CAD build for the part. Positions are in the model's coordinates, mm. Face numbers are marked on the shaded views. Give positions to 0.01 mm unless a question says otherwise; leave off trailing zeros. Write each loop counter-clockwise with the first axis right and the second up, starting at its lowest first coordinate (ties: lowest second). Pieces come first, ordered by that corner, then holes. Notation, with made-up numbers: M -37.75,-23 L 1.25,-23 A19 cw 1.25,-12 Z; hole C 45,-32 d11. An arc over 180 degrees is marked long. One line per question, with ' | ' between items. Start each with the question number.
1. Wall check: L1, parallel to Z at x = -60, y = 0.55; L2, parallel to Z at x = -18, y = 0.95; L3, parallel to Z at x = -71.5, y = 1.75. Give the ranges that are in metal, low to high.
2. Flat gauge pin, fed straight in: pin 1 (5 mm diameter, centred on x = -53, z = -50, fed in from +Y). Where does the tip first touch, or does it go through?
3. Pull direction X, two halves, no side cores. Call the marked faces 1, 2 and 3: released by +X, released by -X, zero draft, split by the parting line, or undercut.
4. Cut at D-D, the plane z = -37.5. Count the separate pieces of the cut face and the enclosed holes in it, then the cut area to 3 significant figures.
5. Cut at B-B, the plane x = -72. Write the cut outline in (y, z), then the cut area to 4 significant figures.
6. Cut at A-A, the plane x = -42. Write the cut outline in (y, z), then the cut area to 3 significant figures.
7. Cut at C-C, the plane y = 2.5. Write the cut outline in (x, z).
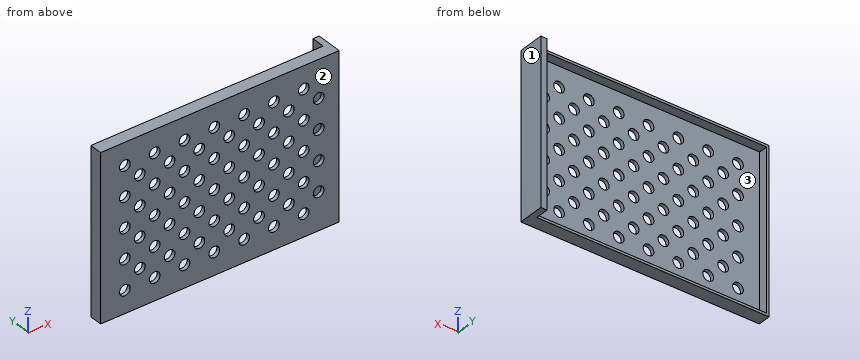
Autodesk Inventor part; units mm, degrees
ref_plane "YZ Plane" through (0, 0, 0) normal (1, 0, 0) x (0, 1, 0)
ref_plane "XZ Plane" through (0, 0, 0) normal (0, 1, 0) x (-1, 0, 0)
ref_plane "XY Plane" through (0, 0, 0) normal (0, 0, 1) x (1, 0, 0)
sketch "Sketch1" plane through (0, 0, 0) normal (0, 1, 0) x (-1, 0, 0)
  line L0 (0, 0) -> (91.5, 0)
  line L1 (91.5, 0) -> (91.5, -63)
  line L2 (91.5, -63) -> (0, -63)
  circle A0 centre (84, -7.5) radius 2.15
  circle A1 centre (84, -19.5) radius 2.15
  circle A2 centre (84, -31.5) radius 2.15
  circle A3 centre (84, -55.5) radius 2.15
  circle A4 centre (84, -43.5) radius 2.15
  circle A5 centre (78, -13.5) radius 2.15
  circle A6 centre (78, -25.5) radius 2.15
  circle A7 centre (78, -37.5) radius 2.15
  circle A8 centre (78, -49.5) radius 2.15
  circle A9 centre (66, -13.5) radius 2.15
  circle A10 centre (66, -25.5) radius 2.15
  circle A11 centre (66, -37.5) radius 2.15
  circle A12 centre (66, -49.5) radius 2.15
  circle A13 centre (72, -31.5) radius 2.15
  circle A14 centre (72, -19.5) radius 2.15
  circle A15 centre (72, -7.5) radius 2.15
  circle A16 centre (72, -55.5) radius 2.15
  circle A17 centre (72, -43.5) radius 2.15
  line L3 (66, -55.5) -> (63, -55.5)
  line L4 (63, -55.5) -> (63, -45.305)
  circle A18 centre (42, -13.5) radius 2.15
  circle A19 centre (42, -25.5) radius 2.15
  circle A20 centre (42, -37.5) radius 2.15
  circle A21 centre (42, -49.5) radius 2.15
  circle A22 centre (48, -31.5) radius 2.15
  circle A23 centre (48, -19.5) radius 2.15
  circle A24 centre (48, -7.5) radius 2.15
  circle A25 centre (48, -55.5) radius 2.15
  circle A26 centre (48, -43.5) radius 2.15
  circle A27 centre (54, -37.5) radius 2.15
  circle A28 centre (60, -31.5) radius 2.15
  circle A29 centre (54, -25.5) radius 2.15
  circle A30 centre (60, -19.5) radius 2.15
  circle A31 centre (54, -13.5) radius 2.15
  circle A32 centre (60, -7.5) radius 2.15
  circle A33 centre (60, -43.5) radius 2.15
  circle A34 centre (54, -49.5) radius 2.15
  circle A35 centre (60, -55.5) radius 2.15
  line L5 (42, -55.5) -> (39, -55.5)
  line L6 (39, -55.5) -> (39, -51.65)
  circle A36 centre (6, -37.5) radius 2.15
  circle A37 centre (12, -31.5) radius 2.15
  circle A38 centre (6, -25.5) radius 2.15
  circle A39 centre (12, -19.5) radius 2.15
  circle A40 centre (6, -13.5) radius 2.15
  circle A41 centre (12, -7.5) radius 2.15
  circle A42 centre (12, -43.5) radius 2.15
  circle A43 centre (6, -49.5) radius 2.15
  circle A44 centre (12, -55.5) radius 2.15
  line L7 (12, -55.5) -> (15, -55.5)
  line L8 (15, -55.5) -> (15, -45.305)
  circle A45 centre (36, -43.5) radius 2.15
  circle A46 centre (30, -49.5) radius 2.15
  circle A47 centre (24, -55.5) radius 2.15
  circle A48 centre (24, -43.5) radius 2.15
  circle A49 centre (36, -55.5) radius 2.15
  circle A50 centre (36, -7.5) radius 2.15
  circle A51 centre (30, -25.5) radius 2.15
  circle A52 centre (30, -13.5) radius 2.15
  circle A53 centre (18, -25.5) radius 2.15
  circle A54 centre (24, -19.5) radius 2.15
  circle A55 centre (18, -13.5) radius 2.15
  circle A56 centre (24, -7.5) radius 2.15
  circle A57 centre (36, -19.5) radius 2.15
  circle A58 centre (36, -31.5) radius 2.15
  circle A59 centre (30, -37.5) radius 2.15
  circle A60 centre (24, -31.5) radius 2.15
  circle A61 centre (18, -49.5) radius 2.15
  circle A62 centre (18, -37.5) radius 2.15
  line L9 (36, -55.5) -> (39, -55.5)
  line L10 (0, 0) -> (0, -63)
  dimension "d0" = 91.5
  dimension "d1" = 63
  dimension "d2" = 4.3
  dimension "d3" = 7.5
  dimension "d4" = 7.5
  dimension "d11" = 4.3
  dimension "d17" = 3
  dimension "d18" = 3
extrude "Extrusion1" add sketch "Sketch1" along normal blind 1.5
sketch "Sketch2" plane through (0, 1.5, 0) normal (0, 1, 0) x (1, 0, 0)
  line L0 (3, 0) -> (3, -3)
  line L1 (3, -3) -> (-94.5, -3)
  line L2 (-94.5, -3) -> (-94.5, 66)
  line L3 (-94.5, 66) -> (3, 66)
  line L4 (3, 66) -> (3, 0)
  line L5 (-91.5, 63) -> (-91.5, 0)
  line L6 (0, 63) -> (-91.5, 63)
  line L7 (-91.5, 0) -> (0, 0)
  line L8 (0, 0) -> (0, 63)
  line L9 (0, 63) -> (-91.5, 63)
  line L10 (-91.5, 63) -> (-91.5, 0)
  dimension "d30" = 97.5
  dimension "d31" = 69
  dimension "d32" = 97.5
extrude "Extrusion2" add sketch "Sketch2" along normal blind 3.612 and the other way blind 1.5
sketch "Sketch5" plane through (0, 1.5, 0) normal (0, 1, 0) x (1, 0, 0)
  point P0 (0, 0)
sketch "Sketch6" plane through (0, 5.112, 0) normal (0, 1, 0) x (1, 0, 0)
  line L0 (0, 0) -> (0, 63)
  line L1 (3, 66) -> (3, -3)
  line L2 (0, 0) -> (3, 0)
  line L3 (3, 0) -> (3, 63)
  line L4 (3, 63) -> (0, 63)
  line L5 (0, 63) -> (0, 0)
extrude "Extrusion3" add sketch "Sketch6" along normal blind 5.388
sketch "Sketch7" plane through (-91.5, 1.5, -63) normal (0, 0, 1) x (1, 0, 0)
  point P0 (91.5, -1.5)
sketch "Sketch8" plane through (-91.5, 1.5, -63) normal (0, 0, 1) x (1, 0, 0)
  line L0 (91.5, 0) -> (0, 0)
  line L1 (0, 3.612) -> (91.5, 3.612)
  line L2 (0, 0) -> (91.5, 0)
  line L3 (91.5, 0) -> (91.5, 3.612)
  line L4 (91.5, 3.612) -> (0, 3.612)
  line L5 (0, 3.612) -> (0, 0)
  point P0 (91.5, -1.5)
extrude "Extrusion4" cut sketch "Sketch8" against normal blind 0.5
sketch "Sketch9" plane through (0, 1.5, 0) normal (0, 0, -1) x (-1, 0, 0)
  line L0 (0, 3.612) -> (91.5, 3.612)
  line L1 (91.5, 0) -> (0, 0)
  line L2 (91.5, 3.612) -> (0, 3.612)
  line L3 (0, 3.612) -> (0, 0)
  line L4 (0, 0) -> (91.5, 0)
  line L5 (91.5, 0) -> (91.5, 3.612)
  point P0 (0, -1.5)
extrude "Extrusion5" cut sketch "Sketch9" against normal blind 0.5
sketch "Sketch10" plane through (-91.5, 1.5, -63.5) normal (1, 0, 0) x (0, 0, -1)
  line L0 (0, 0) -> (0, 3.612)
  line L1 (0, 0) -> (-64, 0)
  line L2 (0, 3.612) -> (-64, 3.612)
  line L3 (-64, 3.612) -> (-64, 0)
  line L4 (-64, 0) -> (0, 0)
  line L5 (0, 0) -> (0, 3.612)
  point P0 (-63.5, -1.5)
extrude "Extrusion6" cut sketch "Sketch10" against normal blind 0.5
sketch "Sketch11" plane through (3, 5.112, -63) normal (0, 0, -1) x (-1, 0, 0)
  line L0 (0, 5.388) -> (3, 5.388)
  line L1 (0, 0) -> (0, 5.388)
  line L2 (3, 5.388) -> (0, 5.388)
  line L3 (0, 5.388) -> (0, 0)
  line L4 (0, 0) -> (3, 0)
  line L5 (3, 0) -> (3, 5.388)
  point P0 (3, -5.112)
extrude "Extrusion7" add sketch "Sketch11" along normal blind 3
sketch "Sketch12" plane through (0, 5.112, 0) normal (0, 0, 1) x (1, 0, 0)
  line L0 (0, 5.388) -> (3, 5.388)
  line L1 (-94.5, 0) -> (3, 0)
  line L2 (0, 5.388) -> (3, 5.388)
  line L3 (3, 5.388) -> (3, 0)
  line L4 (3, 0) -> (0, 0)
  line L5 (0, 0) -> (0, 5.388)
  point P0 (0, -5.112)
extrude "Extrusion8" add sketch "Sketch12" along normal blind 3
sketch "Sketch13" plane through (0, 0, 0) normal (0, -1, 0) x (1, 0, 0)
  line L0 (-94.5, 3) -> (0, 3)
  line L1 (-94.5, 3) -> (-93.75, 3)
  line L2 (-93.75, 1.5) -> (2.25, 1.5)
  line L3 (2.25, 1.5) -> (2.25, -64.5)
  line L4 (2.25, -64.5) -> (-93.75, -64.5)
  line L5 (-93.75, -64.5) -> (-93.75, 1.5)
  line L6 (3, -66) -> (3, 3)
  line L7 (-94.5, 3) -> (3, 3)
  line L8 (3, 3) -> (3, -66)
  line L9 (3, -66) -> (-94.5, -66)
  line L10 (-94.5, -66) -> (-94.5, 3)
  point P0 (0, 0)
  dimension "d45" = 0.75
  dimension "d46" = 1.5
  dimension "d47" = 96
  dimension "d48" = 66
extrude "Extrusion9" cut sketch "Sketch13" against normal through all
sketch "Sketch14" plane through (-93.75, 0, -64.5) normal (-1, 0, 0) x (0, 0, 1)
  line L0 (0, 5.112) -> (66, 5.112)
  line L1 (0, 0) -> (0, 5.112)
  line L2 (66, 5.112) -> (0, 5.112)
  line L3 (0, 5.112) -> (0, 1.5)
  line L4 (0, 1.5) -> (66, 1.5)
  line L5 (66, 1.5) -> (66, 5.112)
  point P0 (64.5, 0)
extrude "Extrusion10" cut sketch "Sketch14" against normal through all
sketch "Sketch15" plane through (0, 10.5, 1.5) normal (0, 0, 1) x (1, 0, 0)
  line L0 (2.25, -5.388) -> (2.25, 0)
  line L1 (0, -5.388) -> (0, 0)
  line L2 (2.25, -5.388) -> (0, -5.388)
  line L3 (0, -5.388) -> (0, 0)
  line L4 (0, 0) -> (2.25, 0)
  line L5 (2.25, 0) -> (2.25, -5.388)
  point P0 (0, -10.5)
extrude "Extrusion11" cut sketch "Sketch15" against normal through all
sketch "Sketch16" plane through (0, 1.5, 0) normal (0, 1, 0) x (1, 0, 0)
  line L0 (2.25, 64.5) -> (2.25, -1.5)
  line L1 (2.25, -1.5) -> (-0.75, -1.5)
  line L2 (-0.75, -1.5) -> (-0.75, 3.5)
  line L3 (-0.75, 3.5) -> (2.25, 3.5)
  line L4 (2.25, 3.5) -> (2.25, -1.5)
  line L5 (2.25, 64.5) -> (-0.75, 64.5)
  line L6 (-0.75, 64.5) -> (-0.75, 59.5)
  line L7 (-0.75, 59.5) -> (2.25, 59.5)
  line L8 (2.25, 59.5) -> (2.25, 64.5)
  line L9 (2.25, 3.5) -> (-0.75, 3.5)
  line L10 (-0.75, 3.5) -> (-0.75, 59.5)
  line L11 (-0.75, 59.5) -> (2.25, 59.5)
  line L12 (2.25, 59.5) -> (2.25, 3.5)
  point P0 (0, 0)
  dimension "d55" = 3
  dimension "d56" = 5
  dimension "d57" = 3
  dimension "d58" = 5
extrude "Extrusion12" add sketch "Sketch16" along normal blind 9
sketch "Sketch17" plane through (0, 1.5, 0) normal (0, 1, 0) x (1, 0, 0)
  line L0 (-0.75, -1.5) -> (-93.75, -1.5)
  line L1 (-0.75, -1.5) -> (-0.75, 0)
  line L2 (-0.75, -1.5) -> (-0.75, 64.5)
  line L3 (-93.75, -1.5) -> (-93.75, 64.5)
  line L4 (-93.75, -1.5) -> (-93.75, 64.5)
  line L5 (-93.75, 64.5) -> (-0.75, 64.5)
  line L6 (-93.75, 64.5) -> (-0.75, 64.5)
  line L7 (-0.75, 64.5) -> (-0.75, 63)
  line L8 (-92.25, 63) -> (-0.75, 63)
  line L9 (-0.75, 0) -> (-92.25, 0)
  line L10 (-92.25, 0) -> (-92.25, 63)
  point P0 (0, 0)
  dimension "d61" = 1.5
extrude "Extrusion13" add sketch "Sketch17" along normal blind 3.65 contours L0 L3 L5 L2 L8 L10 L9 L1
sketch "Sketch18" plane through (-0.75, 1.5, 0) normal (0, 0, -1) x (-1, 0, 0)
  line L0 (91.5, 0) -> (91.5, 3.65)
  line L1 (0, 0) -> (0, 3.65)
  line L2 (91.5, 3.65) -> (0, 3.65)
  line L3 (0, 3.65) -> (0, 0)
  line L4 (0, 0) -> (91.5, 0)
  line L5 (91.5, 0) -> (91.5, 3.65)
  point P0 (-0.75, -1.5)
extrude "Extrusion14" cut sketch "Sketch18" against normal blind 0.5
sketch "Sketch19" plane through (-92.25, 1.5, -63) normal (0, 0, 1) x (1, 0, 0)
  line L0 (91.5, 0) -> (0, 0)
  line L1 (0, 0) -> (0, 3.65)
  line L2 (91.5, 0) -> (0, 0)
  line L3 (0, 0) -> (0, 3.65)
  line L4 (0, 3.65) -> (91.5, 3.65)
  line L5 (91.5, 3.65) -> (91.5, 0)
  point P0 (92.25, -1.5)
extrude "Extrusion15" cut sketch "Sketch19" against normal blind 0.5
sketch "Sketch20" plane through (-92.25, 1.5, 0.5) normal (1, 0, 0) x (0, 0, -1)
  line L0 (64, 0) -> (64, 3.65)
  line L1 (64, 0) -> (0, 0)
  line L2 (0, 0) -> (0, 3.65)
  line L3 (0, 3.65) -> (64, 3.65)
  line L4 (64, 3.65) -> (64, 0)
  point P0 (0.5, -1.5)
extrude "Extrusion16" cut sketch "Sketch20" against normal blind 0.5
sketch "Sketch21" plane through (-0.75, 10.5, -64.5) normal (-1, 0, 0) x (0, 0, 1)
  line L0 (1, -5.35) -> (1, -9)
  line L1 (1, -9) -> (1, -5.35)
  line L2 (0, -5.35) -> (1, -5.35)
  line L3 (1, -5.35) -> (0, -5.35)
  line L4 (0, -5.35) -> (0, 0)
  line L5 (66, -5.35) -> (66, 0)
  line L6 (0, 0) -> (66, 0)
  line L7 (65, -5.35) -> (66, -5.35)
  line L8 (66, -5.4693) -> (65, -5.35)
  line L9 (65, -9) -> (65, -5.35)
  line L10 (65, -5.35) -> (65, -9)
  line L11 (65, -5.35) -> (66, -5.35)
  line L12 (66, -5.35) -> (66, 0)
  line L13 (65, -9) -> (1, -9)
  line L14 (65, -9) -> (1, -9)
  line L15 (1, -9) -> (1, -5.35)
  line L16 (1, -5.35) -> (0, -5.35)
  point P0 (64.5, -10.5)
extrude "Extrusion17" cut sketch "Sketch21" against normal blind 0.5
properties part number "RaspPiCaseTop"
Here are the results:
1) L1: -64.5 to -57.65, -53.35 to -45.65, -41.35 to -33.65, -29.35 to -21.65, -17.35 to -9.65, -5.35 to 1.5 | L2: -64.5 to -51.65, -47.35 to -39.65, -35.35 to -27.65, -23.35 to -15.65, -11.35 to 1.5 | L3: -64.5 to -63.5, 0.5 to 1.5
2) pin 1: y = 1.5
3) face 1: released by +X | face 2: zero draft | face 3: undercut
4) separate pieces: 8 | enclosed holes: 0 | area: 125 mm^2
5) outline: M 0,-64.5 L 5.15,-64.5 L 5.15,-63.5 L 1.5,-63.5 L 1.5,-57.65 L 0,-57.65 Z; M 0,-53.35 L 1.5,-53.35 L 1.5,-45.65 L 0,-45.65 Z; M 0,-41.35 L 1.5,-41.35 L 1.5,-33.65 L 0,-33.65 Z; M 0,-29.35 L 1.5,-29.35 L 1.5,-21.65 L 0,-21.65 Z; M 0,-17.35 L 1.5,-17.35 L 1.5,-9.65 L 0,-9.65 Z; M 0,-5.35 L 1.5,-5.35 L 1.5,0.5 L 5.15,0.5 L 5.15,1.5 L 0,1.5 Z | area: 74.05 mm^2
6) outline: M 0,-64.5 L 5.15,-64.5 L 5.15,-63.5 L 1.5,-63.5 L 1.5,-51.65 L 0,-51.65 Z; M 0,-47.35 L 1.5,-47.35 L 1.5,-39.65 L 0,-39.65 Z; M 0,-35.35 L 1.5,-35.35 L 1.5,-27.65 L 0,-27.65 Z; M 0,-23.35 L 1.5,-23.35 L 1.5,-15.65 L 0,-15.65 Z; M 0,-11.35 L 1.5,-11.35 L 1.5,0.5 L 5.15,0.5 L 5.15,1.5 L 0,1.5 Z | area: 80.5 mm^2
7) outline: M -93.75,-64.5 L 2.25,-64.5 L 2.25,1.5 L -93.75,1.5 Z; hole M -92.75,-63.5 L -0.25,-63.5 L -0.25,0.5 L -92.75,0.5 Z
